from build123d import *

# Parameters (mm, degrees)
F0_R      = 13
F0_R_2    = 9.5
F1_DEPTH  = 17.4
F2_R      = 14.2
F3_R      = 14.2
F4_DEPTH  = 7.5
F5_R      = 9.5
F6_DEPTH  = 25
F9_R      = 16.7063841851
F9_R_2    = 15.935
F10_DEPTH = 25


with BuildPart() as f1:
    # F0 (on Top) → F1 (new body)
    with BuildSketch(Plane.XY):
        Circle(F0_R)
        Circle(F0_R_2, mode=Mode.SUBTRACT)
    extrude(amount=F1_DEPTH)

    # F2 (on Top) + F3 (on face) → F4 (join)
    with BuildSketch(Plane.XY):
        Circle(F2_R)
    with BuildSketch(Plane.XY):
        Polygon((11.6155659336, -11.648343784), (15.8955445957, 4.2352032858), (4.2799786621, 15.8835470698), (-11.6155659336, 11.648343784), (-15.8955445957, -4.2352032858), (-4.2799786621, -15.8835470698), align=None)
        Circle(F3_R, mode=Mode.SUBTRACT)
    extrude(amount=F4_DEPTH)

    # F5 (on face) → F6 (cut)
    with BuildSketch(Plane.XY):
        Circle(F5_R)
    extrude(amount=F6_DEPTH, mode=Mode.SUBTRACT)

    # F7 (on face) → F8 (revolve, cut)
    with BuildSketch(Plane(origin=(-10.0877616289, -10.0593751778, 0), x_dir=(0.7061097972, -0.7081023614, 0), z_dir=(-0.7081023614, -0.7061097972, 0))):
        with BuildLine():
            ThreePointArc((-5.4935941607, 0), (-7.2307127812, 0.6945951349), (-8.2250423231, 2.2793198004))
            Line((-8.2250423231, 2.2793198004), (-8.2250423231, 0))
            Line((-8.2250423231, 0), (-5.4935941607, 0))
        make_face()
        with BuildLine():
            Line((-8.2250423231, 7.5), (-8.2250423231, 5.0454880111))
            ThreePointArc((-8.2250423231, 5.0454880111), (-7.2682177888, 6.7453516877), (-5.4694527589, 7.5))
            Line((-5.4694527589, 7.5), (-8.2250423231, 7.5))
        make_face()
    revolve(axis=Axis((0, 0, 0), (0, 0, -1)), mode=Mode.SUBTRACT)

    # F9 (on face) → F10 (cut)
    with BuildSketch(Plane(origin=(0, 0, 0), x_dir=(1, 0, 0), z_dir=(0, 0, -1))):
        Circle(F9_R)
        Circle(F9_R_2, mode=Mode.SUBTRACT)
    extrude(amount=-F10_DEPTH, mode=Mode.SUBTRACT)


solid = f1.part
The model under review builds one solid part; all positions refer to its coordinate system, in mm. A direction names the side the tool comes from. Round coordinates to 2 decimals unless told otherwise and drop trailing zeros. Write each loop counter-clockwise with the first axis right and the second up, starting at its lowest first coordinate (ties: lowest second). Pieces come first, ordered by that corner, then holes. Notation, with made-up numbers: M 80.25,79 L 102.25,79 A23 ccw 102.25,112 Z; hole C -27,78.5 d5. An arc over 180 degrees is marked long. Answer as CSV lines item,"result". Start each with the question number.
Q1. Clearance check with flat-ended pins moving along their axes: P1, Ø2, axis at x = 6, z = 6.5, coming from the +Y side; P2, Ø8, axis at y = 7, z = 15, coming from the +X side; P3, Ø2, axis at x = -12, z = 5.5, coming from the +Y side. State where each tip first meets the part, or that it passes through.
Q2. Consider section D-D, the plane z = 13.25. Give the boundary of the cut face in (x, y).
Q3. Consider section B-B, the plane x = 0. Give the boundary of the cut face in (y, z).
Q4. Consider section C-C, the plane y = 0. Give the boundary of the cut face in (x, z).
Q5. Wall thickness on line 1 along Z through (x, y) = (-10, -10); line 2 along Y through (x, z) = (-4, 11.5); line 3 along X through (y, z) = (-1, 13): over which ranges is each line inside the solid? List them lowest first.
Q6. Tool access review of faces 4 (the face through (10.158, 9.989, 3.698)), 5 (the face through (-0.1, -13.4, 7.5)): name each direction out of +Z, -Z, +X, -X, +Y, -Y from which nothing blocks a thin tool from reaching the whole face with its end or side.
Q7. Consider section A-A, the plane z = 2.5. Give the boundary of the cut face in (x, y) (3 decimals).
Q8. The part is to be moulded in two halves that separate along Y. For faces 1 (the face through (-10.316, -7.91, 12.381)), 2 (the face through (4.38, -8.43, 8.58)), 3 (the face through (-11.261, 11.274, 3.694)), say which applies: +Y half, -Y half, draft (parallel to the pull), parting line (faces both ways), or undercut.
Result set:
1,P1,"stops at y = 15.13"
1,P2,"stops at x = 12.65"
1,P3,"stops at y = 11.53"
2,outline,"C 0,0 d26; hole C 0,0 d19"
3,outline,"M -14.74,0 L -9.5,0 L -9.5,17.4 L -13,17.4 L -13,7.5 L -14.74,7.5 Z; M 9.5,0 L 14.74,0 L 14.74,7.5 L 13,7.5 L 13,17.4 L 9.5,17.4 Z"
4,outline,"M -14.75,0 L -9.5,0 L -9.5,17.4 L -13,17.4 L -13,7.5 L -14.75,7.5 Z; M 9.5,0 L 14.75,0 L 14.75,7.5 L 13,7.5 L 13,17.4 L 9.5,17.4 Z"
5,line 1,"z = 0 to 7.5"
5,line 2,"y = -12.37 to -8.62, 8.62 to 12.37"
5,line 3,"x = -12.96 to -9.45, 9.45 to 12.96"
6,face 4,"+Z, -Z, +X, +Y"
6,face 5,"+Z"
7,outline,"M -15.613,-3.187 A15.935 ccw -15.129,-5.004 L -5.047,-15.115 A15.935 ccw -3.231,-15.604 L 10.566,-11.928 A15.935 ccw 11.898,-10.6 L 15.613,3.187 A15.935 ccw 15.129,5.004 L 5.047,15.115 A15.935 ccw 3.231,15.604 L -10.566,11.928 A15.935 ccw -11.898,10.6 Z; hole C 0,0 d19"
8,face 1,"parting line"
8,face 2,"undercut"
8,face 3,"+Y half"
